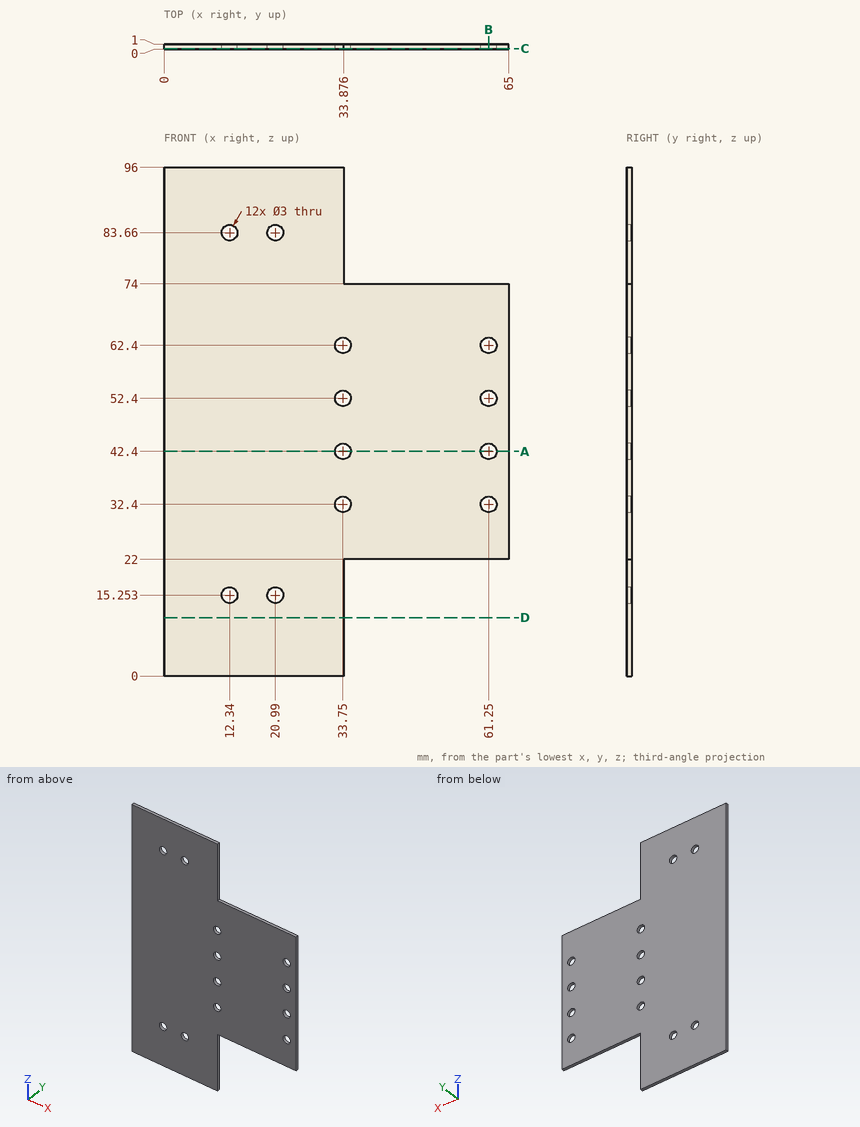
Geometry check sheet. Reference: drawing and pictorial views, mm from the part's lowest x, y, z. Give positions to 0.01 mm unless a question says otherwise; leave off trailing zeros. Write each loop counter-clockwise with the first axis right and the second up, starting at its lowest first coordinate (ties: lowest second). Pieces come first, ordered by that corner, then holes. Notation, with made-up numbers: M 11,82.5 L 37,82.5 A13 cw 37,92.5 Z; hole C 40,-5 d8. An arc over 180 degrees is marked long. Use CSV: the item, a comma, the result in double quotes.
1) Cross-section at C-C (y = 0.15). State how many separate pieces and enclosed holes the cut face has, plus the area to 3 significant figures.
Final values:
separate pieces,"1"
enclosed holes,"12"
area,"4,790 mm²"
2) Cross-section at A-A (z = 42.4). Enter the section's corners in (x, y).
Final values:
outline,"M 0,0 L 32.25,0 L 32.25,1 L 0,1 Z; M 35.25,0 L 59.75,0 L 59.75,1 L 35.25,1 Z; M 62.75,0 L 65,0 L 65,1 L 62.75,1 Z"
3) Material ranges on line 1 along X through (y, z) = (0.7, 32.4); line 2 along X through (y, z) = (0.65, 82.5) (1 decimal); line 3 along Z through (x, y) = (39.5, 0.45), recorded low to high.
Final values:
line 1,"0 to 32.25, 35.25 to 59.75, 62.75 to 65"
line 2,"0 to 11.4, 13.3 to 20, 21.9 to 33.9"
line 3,"22 to 74"
4) Cross-section at B-B (x = 61.25). Enter the section's corners in (y, z).
Final values:
outline,"M 0,22 L 1,22 L 1,30.9 L 0,30.9 Z; M 0,33.9 L 1,33.9 L 1,40.9 L 0,40.9 Z; M 0,43.9 L 1,43.9 L 1,50.9 L 0,50.9 Z; M 0,53.9 L 1,53.9 L 1,60.9 L 0,60.9 Z; M 0,63.9 L 1,63.9 L 1,74 L 0,74 Z"
5) Cross-section at D-D (z = 11). Enter the section's corners in (x, y).
Final values:
outline,"M 0,0 L 33.88,0 L 33.88,1 L 0,1 Z"
6) Go/stop test with a flat-tipped pin: pin 1 Ø5 at (x, z) = (48, 31) entering from -Y. Record where the tip stops, or that it passes through.
Final values:
pin 1,"y = 0"
